For this review, use the dimensioned drawing (mm, ordinates from the lowest corner) and the shaded views. A direction names the side the tool comes from. Round coordinates to 2 decimals unless told otherwise and drop trailing zeros. Loops run counter-clockwise (first coordinate to the right, second up) from the corner with the lowest first, then second, coordinate; pieces in that order, holes last. Notation, with made-up numbers: M 66.5,68 L 89.5,68 A14 cw 89.5,95 Z; hole C 4.25,76 d1. An arc over 180 degrees is marked long. Answer as a JSON object with one key per item and string values. Group by question number.
Item 1: To check wall thickness, follow line 1 (X direction, y = 23.25, z = 29); line 2 (X direction, y = 11, z = 19.5); line 3 (Z direction, x = 29, y = 0.8). State the ranges of each line that lie inside material, in increasing order.
Item 2: Consider section C-C (y = 16). Give the boundary of the cut face in (x, z), and give its area (3 significant figures).
Item 3: Consider section D-D (z = 6.5). Give the boundary of the cut face in (x, y).
Item 4: Insertion check: P1, Ø0.9, axis at y = 1.5, z = 7, coming from the +X side; P2, Ø4, axis at x = 26, y = 20, coming from the +Z side; P3, Ø4, axis at y = 7.5, z = 31.5, coming from the +X side; P4, Ø2, axis at x = 29, z = 54, coming from the -Y side. Each pin has a flat end and moves straight along its axis. Give the tip position at first contact, or say it passes through.
Item 5: Consider section A-A (z = 29). State how many separate pieces and enclosed holes the cut face has, and give its area (3 significant figures).
Item 6: The part is to be moulded in two halves that separate along Z. For the marked faces 3, 4, 5 and 6, say which applies: +Z half, -Z half, draft (parallel to the pull), parting line (faces both ways), or undercut.
Item 7: Tool access review of the marked faces 1 and 2: name each direction out of +Z, -Z, +X, -X, +Y, -Y from which nothing blocks a thin tool from reaching the whole face with its end or side.
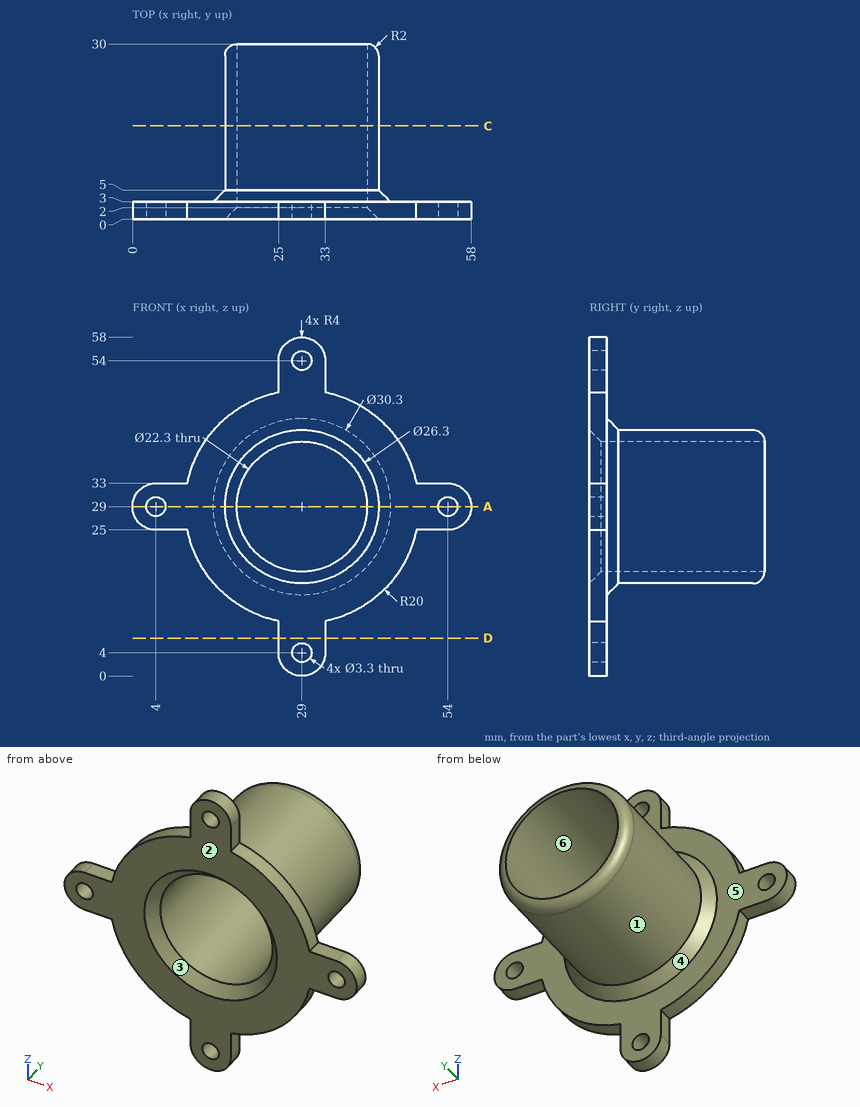
Geometry results:
{
 "1": {"line 1": "x = 15.85 to 17.85, 40.15 to 42.15", "line 2": "x = 19.91 to 23.16, 34.84 to 38.09", "line 3": "z = 0 to 2.35, 5.65 to 16.65, 41.35 to 52.35, 55.65 to 58"},
 "2": {"outline": "C 29,29 d26.3; hole C 29,29 d22.3", "area": "153 mm^2"},
 "3": {"outline": "M 25,0 L 33,0 L 33,3 L 25,3 Z"},
 "4": {"P1": "stops at x = 33", "P2": "stops at z = 42.11", "P3": "stops at x = 42.14", "P4": "passes through"},
 "5": {"separate pieces": "4", "enclosed holes": "0", "area": "194 mm^2"},
 "6": {"face 3": "undercut", "face 4": "parting line", "face 5": "draft", "face 6": "undercut"},
 "7": {"face 1": "+Y", "face 2": "+Z, -Z, +X, -X, -Y"}
}
